The model under review builds one solid part; all positions refer to its coordinate system, in mm. Face numbers are marked on the shaded views. A direction names the side the tool comes from. Round coordinates to 2 decimals unless told otherwise and drop trailing zeros. Loops run counter-clockwise (first coordinate to the right, second up) from the corner with the lowest first, then second, coordinate; pieces in that order, holes last. Notation, with made-up numbers: M 47,5 L 72,5 A23 ccw 72,23 Z; hole C -27,44 d11. An arc over 180 degrees is marked long. Return JSON: item names as keys, results as strings. Group by question number.
Q1. To check wall thickness, follow line 1 along Y through (x, z) = (-11, -56); line 2 along Z through (x, y) = (58, 458); line 3 along Y through (x, z) = (57, -96). State the ranges of each line that lie inside material, in increasing order.
Q2. For the marked faces 5, 6, 7, 8 and 9, list the 3-axis set-ups (+Z, -Z, +X, -X, +Y, -Y) from which the entire face can be reached by the end or side of a thin tool; tool diameter is ignored.
Q3. Draft analysis for pull direction Y (two halves, no side actions). For the marked faces 1, 2, 3 and 4, state which applies: pulls with the +Y half, pulls with the -Y half, needs draft (parallel to the pull), parting line crosses it, or undercut.
Q4. Consider section A-A (y = -72.5). State the section outline as (x, z) points.
Q5. Consider section B-B (y = 233.5). State the section outline as (x, z) points, and give its area (3 significant figures).
Q6. Clearance check with flat-ended pins moving along their axes: pin 1 Ø3 at (x, y) = (-85.5, 216) entering from -Z; pin 2 Ø17 at (x, z) = (109.5, -0.5) entering from -Y; pin 3 Ø2 at (x, y) = (40, 135.5) entering from -Z; pin 4 Ø20 at (x, z) = (113, 8) entering from +Y. State where each tip first meets the part, or that it passes through.
from build123d import *

# Parameters (mm, degrees)
F0_R          = 62.5146568837
F1_DEPTH      = 93.62484
F1_DEPTH_BACK = 67.66725
F2_R          = 78.9516087872
F3_DEPTH      = 97.98912
F4_R          = 54.5557763687
F5_DEPTH      = 40.02087
F6_R          = 62.0868515923
F7_DEPTH      = 64.06144
F8_R          = 98.3447043225
F9_DEPTH      = 164.96345
F11_DEPTH     = 313.96558
F12_W         = 63.6207908392
F12_H         = 54.3301105499
F13_DEPTH     = 25.4
F15_DEPTH     = 76.2
F17_DEPTH     = 203.2
F18_W         = 123.2421994209
F18_H         = 87.3634591699
F18_R         = 9.0836409793
F20_DEPTH     = 7.62
F22_DEPTH     = 12.18293


with BuildPart() as f1:
    # F0 (on Front) → F1 (new body, two sides)
    with BuildSketch(Plane.XZ) as f1_sk:
        Circle(F0_R)
    extrude(amount=F1_DEPTH)
    extrude(f1_sk.sketch, amount=-F1_DEPTH_BACK)

    # F2 (on face) → F3 (join)
    with BuildSketch(Plane.XZ.offset(93.62484)):
        Circle(F2_R)
    extrude(amount=-F3_DEPTH)

    # F4 (on face) → F5 (join)
    with BuildSketch(Plane(origin=(0, 67.66725, 0), x_dir=(-1, 0, 0), z_dir=(0, 1, 0))):
        Circle(F4_R)
    extrude(amount=F5_DEPTH)

    # F6 (on face) → F7 (join)
    with BuildSketch(Plane(origin=(0, 107.68812, 0), x_dir=(-1, 0, 0), z_dir=(0, 1, 0))):
        Circle(F6_R)
    extrude(amount=F7_DEPTH)

    # F8 (on face) → F9 (join)
    with BuildSketch(Plane(origin=(0, 171.74956, 0), x_dir=(-1, 0, 0), z_dir=(0, 1, 0))):
        Circle(F8_R)
    extrude(amount=F9_DEPTH)

    # F10 (on face) → F11 (join)
    with BuildSketch(Plane(origin=(0, 336.71301, 0), x_dir=(-1, 0, 0), z_dir=(0, 1, 0))):
        with BuildLine():
            add(Edge.make_bspline(
                [(0, -91.3981422782), (-40.1217959726, -92.0347084682), (-83.3063936827, -46.5341806253), (-83.5479795933, 0)],
                knots=[0.748537523, 0.748537523, 0.748537523, 0.748537523, 1, 1, 1, 1], degree=3))
            Line((-83.5479795933, 0), (-104.587353766, 0))
            Line((-104.587353766, 0), (-104.587353766, -98.3447043225))
            Line((-104.587353766, -98.3447043225), (0, -98.3447043225))
            Line((0, -98.3447043225), (0, -91.3981422782))
        make_face()
        with BuildLine():
            Line((-104.587353766, 0), (-83.5479795933, 0))
            add(Edge.make_bspline(
                [(-83.5479795933, 0), (-83.7916500228, 46.9356998238), (-40.34804577, 94.9229670887), (0, 94.285428524)],
                knots=[0, 0, 0, 0, 0.2536322157, 0.2536322157, 0.2536322157, 0.2536322157], degree=3))
            Line((0, 94.285428524), (0, 98.3447043225))
            Line((0, 98.3447043225), (-104.587353766, 98.3447043225))
            Line((-104.587353766, 98.3447043225), (-104.587353766, 0))
        make_face()
        with BuildLine():
            Line((0, 98.3447043225), (0, 94.285428524))
            add(Edge.make_bspline(
                [(0, 94.285428524), (39.5484573968, 93.6605242373), (76.1228316851, 46.3189404004), (75.8891776204, 0)],
                knots=[0.2536322157, 0.2536322157, 0.2536322157, 0.2536322157, 0.5022381317, 0.5022381317, 0.5022381317, 0.5022381317], degree=3))
            Line((75.8891776204, 0), (104.587353766, 0))
            Line((104.587353766, 0), (104.587353766, 98.3447043225))
            Line((104.587353766, 98.3447043225), (0, 98.3447043225))
        make_face()
        with BuildLine():
            Line((104.587353766, 0), (75.8891776204, 0))
            add(Edge.make_bspline(
                [(75.8891776204, 0), (75.6576913596, -45.8892009211), (39.2980059924, -90.7746462122), (0, -91.3981422782)],
                knots=[0.5022381317, 0.5022381317, 0.5022381317, 0.5022381317, 0.748537523, 0.748537523, 0.748537523, 0.748537523], degree=3))
            Line((0, -91.3981422782), (0, -98.3447043225))
            Line((0, -98.3447043225), (104.587353766, -98.3447043225))
            Line((104.587353766, -98.3447043225), (104.587353766, 0))
        make_face()
    extrude(amount=F11_DEPTH)

    # F12 (on face) → F13 (join)
    with BuildSketch(Plane.XY.offset(98.3447043225)):
        with Locations((31.8103954196, 536.9567275047)):
            Rectangle(F12_W, F12_H)
        with Locations((-31.8103954196, 536.9567275047)):
            Rectangle(F12_W, F12_H)
        with Locations((31.8103954196, 482.6266169548)):
            Rectangle(F12_W, F12_H)
        with Locations((-31.8103954196, 482.6266169548)):
            Rectangle(F12_W, F12_H)
    extrude(amount=F13_DEPTH)

    # F14 (on face) → F15 (join)
    with BuildSketch(Plane.XZ.offset(93.62484)):
        Polygon((-67.7192732692, 117.2932219539), (-67.7192732692, -117.2932219539), (135.4385465384, 0), align=None)
    extrude(amount=F15_DEPTH)

    # F16 (on face) → F17 (join)
    with BuildSketch(Plane.XZ.offset(169.82484)):
        Polygon((97.5546226371, 133.206090602), (-164.1371697187, 17.8817361593), (66.5825470816, -151.0878267614), align=None)
    extrude(amount=F17_DEPTH)

    # F18 (on face) → F20 (join)
    with BuildSketch(Plane(origin=(-104.587353766, 0, 0), x_dir=(0, -1, 0), z_dir=(-1, 0, 0))):
        with Locations((-559.6050322056, 43.6817295849)):
            Rectangle(F18_W, F18_H)
        with Locations((-615.2921915054, -17.6525395364)):
            Circle(F18_R)
        with BuildLine():
            ThreePointArc((-563.9078745674, -17.6525395364), (-572.3003745079, -9.2600395959), (-580.6928744484, -17.6525395364))
            ThreePointArc((-580.6928744484, -17.6525395364), (-572.3003745079, -26.0450394768), (-563.9078745674, -17.6525395364))
        make_face()
    extrude(amount=F20_DEPTH)

    # F21 (on face) → F22 (cut)
    with BuildSketch(Plane(origin=(-112.207353766, 0, 0), x_dir=(0, -1, 0), z_dir=(-1, 0, 0))):
        Polygon((-572.8379487991, 13.5121122003), (-608.2543730736, 67.1958848834), (-608.2543730736, 13.5121122003), align=None)
        Polygon((-601.2495756149, 71.9198659062), (-601.1453866959, 67.6123201847), (-565.961514646, 14.2810472532), (-506.7166686058, 14.2810472532), (-506.7166686058, 71.9198659062), align=None)
    extrude(amount=-F22_DEPTH, mode=Mode.SUBTRACT)


solid = f1.part
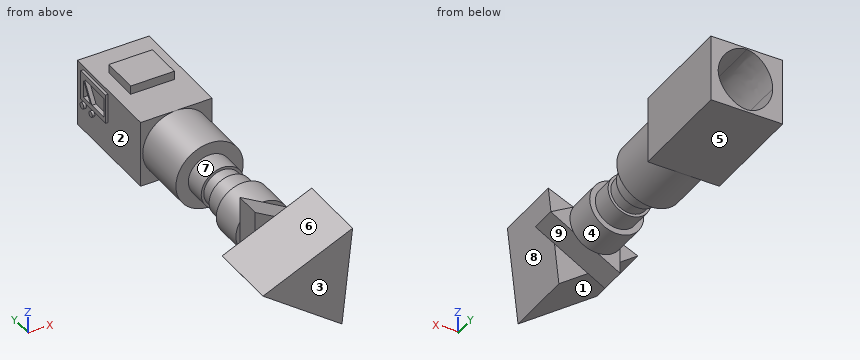
Values:
{
 "1": {"line 1": "y = -373.02 to 67.67, 107.69 to 336.71", "line 2": "z = -98.34 to -61.99, 63.84 to 123.74", "line 3": "y = -373.02 to -169.82, 336.71 to 650.68"},
 "2": {"face 5": "-Z, +X, -X, +Y", "face 6": "+Z, -X, -Y", "face 7": "none", "face 8": "-Z, +X, -Y", "face 9": "-Z, +X"},
 "3": {"face 1": "needs draft", "face 2": "undercut", "face 3": "pulls with the -Y half", "face 4": "undercut"},
 "4": {"outline": "C 0,0 d157.9"},
 "5": {"outline": "C 0,0 d196.69", "area": "30,400 mm2"},
 "6": {"pin 1": "stops at z = -51.14", "pin 2": "stops at y = -169.82", "pin 3": "stops at z = -48.31", "pin 4": "stops at y = 650.68"}
}
